from build123d import *

# Parameters (mm, degrees)
SKETCH2_W              = 45
SKETCH2_H              = 20
BOSS_EXTRUDE1_DEPTH    = 2.54
M1_6_CLEARANCE_HOLE1_D = 1.8
SKETCH6_R              = 8
BOSS_EXTRUDE2_DEPTH    = 12.7


with BuildPart() as part:
    # Sketch2 → Boss-Extrude1 (new body)
    with BuildSketch(Plane(origin=(0, 0, 0), x_dir=(1, 0, 0), z_dir=(0, 1, 0))):
        with Locations((22.5, 10)):
            Rectangle(SKETCH2_W, SKETCH2_H)
    extrude(amount=BOSS_EXTRUDE1_DEPTH)

    # M1.6 Clearance Hole1 (through all)
    with Locations(Plane(origin=(0, 2.54, 0), x_dir=(1, 0, 0), z_dir=(0, 1, 0))):
        with Locations((43.75, 18.75), (1.25, 18.75), (1.25, 1.25), (43.75, 1.25)):
            Hole(M1_6_CLEARANCE_HOLE1_D / 2)

    # Sketch6 → Boss-Extrude2 (add)
    with BuildSketch(Plane(origin=(0, 2.54, 0), x_dir=(1, 0, 0), z_dir=(0, 1, 0))):
        with Locations((9.5, 10)):
            Circle(SKETCH6_R)
        with Locations((35.5, 10)):
            Circle(SKETCH6_R)
    extrude(amount=BOSS_EXTRUDE2_DEPTH)


solid = part.part
Design review of the part built by this model. Coordinates are the model's own, in mm. A direction names the side the tool comes from. Give positions to 0.01 mm unless a question says otherwise; leave off trailing zeros. Loops run counter-clockwise (first coordinate to the right, second up) from the corner with the lowest first, then second, coordinate; pieces in that order, holes last. Notation, with made-up numbers: (3.25, -2.5) - (48.25, -2.5) arc R12 ccw to (48.25, 10.5) - close; hole circle Ø6 at (53, 89). An arc over 180 degrees is marked (long way). Write item = value, one per line.
1) Draft analysis for pull direction Z (two halves, no side actions). For faces 1 (the face through (22, 2.54, -10)), 2 (the face through (7.77, 8.8, -2.19)), 3 (the face through (1.37, 1.25, -19.64)), state which applies: +Z half, -Z half, draft (parallel to the pull), parting line (faces both ways), or undercut.
Result sheet:
face_1 = draft
face_2 = parting line
face_3 = undercut
2) Take a section at C-C on y = 9.75. State the section outline as (x, z) points, and give its area (3 significant figures).
Result sheet:
outline = circle Ø16 at (9.5, -10); circle Ø16 at (35.5, -10)
area = 402 mm2
3) To check wall thickness, follow line 1 (X direction, y = 1.45, z = -18.75); line 2 (Z direction, x = 1.25, y = 2); line 3 (Y direction, x = 18, z = -12.5). State the ranges of each line that lie inside material, in increasing order.
Result sheet:
line_1 = 0 to 0.35, 2.15 to 42.85, 44.65 to 45
line_2 = -20 to -19.65, -17.85 to -2.15, -0.35 to 0
line_3 = 0 to 2.54
4) Take a section at B-B on x = 35.5. State the section outline as (y, z) points, and give its area (3 significant figures).
Result sheet:
outline = (0, -20) - (2.54, -20) - (2.54, -18) - (15.24, -18) - (15.24, -2) - (2.54, -2) - (2.54, 0) - (0, 0) - close
area = 254 mm2
5) Clearance check with flat-ended pins moving along their axes: pin 1 Ø4 at (x, y) = (11, 5) entering from -Z; pin 2 Ø1.5 at (y, z) = (6, -8.5) entering from -X; pin 3 Ø6 at (x, y) = (4.5, 13.5) entering from +Z; pin 4 Ø2 at (x, z) = (38, -2.5) entering from -Y. State where each tip first meets the part, or that it passes through.
Result sheet:
pin_1 = -18
pin_2 = 1.54
pin_3 = -2.25
pin_4 = 0
6) Take a section at D-D on z = -13.5. State the section outline as (x, y) points, and give its area (3 significant figures).
Result sheet:
outline = (0, 0) - (45, 0) - (45, 2.54) - (42.69, 2.54) - (42.69, 15.24) - (28.31, 15.24) - (28.31, 2.54) - (16.69, 2.54) - (16.69, 15.24) - (2.31, 15.24) - (2.31, 2.54) - (0, 2.54) - close
area = 480 mm2
7) Tool access review of faces 4 (the face through (22, 0, -10)), 5 (the face through (29.151, 8.801, -5.132)): name each direction out of +Z, -Z, +X, -X, +Y, -Y from which nothing blocks a thin tool from reaching the whole face with its end or side.
Result sheet:
face_4 = +Z, -Z, +X, -X, -Y
face_5 = +Y
8) Take a section at A-A on z = -18.75. State the section outline as (x, y) points.
Result sheet:
outline = (0, 0) - (0.35, 0) - (0.35, 2.54) - (0, 2.54) - close; (2.15, 0) - (42.85, 0) - (42.85, 2.54) - (2.15, 2.54) - close; (44.65, 0) - (45, 0) - (45, 2.54) - (44.65, 2.54) - close
